Source: CAD feature listing. Evaluate the final solid. Frame: model axes, mm. Face numbers are marked on the shaded views. Give positions to 0.01 mm unless a question says otherwise; leave off trailing zeros. Write each loop counter-clockwise with the first axis right and the second up, starting at its lowest first coordinate (ties: lowest second). Pieces come first, ordered by that corner, then holes. Notation, with made-up numbers: (-3.5, -5.75) - (48.5, -5.75) arc R18 ccw to (48.5, 13.25) - close; hole circle Ø8 at (34, 41). An arc over 180 degrees is marked (long way). One line per question, with ' | ' between items. Start each with the question number.
(1) Section B-B, the plane y = 23.5. Return loops of the section in (x, z).
(2) Ray query, line 1 (X direction, y = 1, z = 0); line 2 (X direction, y = 3.4, z = 0); line 3 (X direction, y = 13, z = 0). Return the intervals inside material, ascending. Write a range as [from, to].
(3) Draft query along X for the marked faces 1, 2, 3 and 4. Return one class per face: +X half, -X half, draft (parallel to the pull), parting line (faces both ways), or undercut.
(4) Pin query (flat end, axial travel): pin 1 (2 mm diameter, centred on y = 5.5, z = 20.5, fed in from -X); pin 2 (12 mm diameter, centred on x = 16, z = -14, fed in from +Y) (3 decimals); pin 3 (6.5 mm diameter, centred on x = 17.5, z = -1.5, fed in from +Y). Return the tip coordinate at first contact, or that it passes through.
(5) Section C-C, the plane y = 5. Return loops of the section in (x, z).
```python
from build123d import *

# Parameters (mm, degrees)
SKETCH1_R           = 25
SKETCH1_R_2         = 1.8
SKETCH1_R_3         = 5.5
BOSS_EXTRUDE1_DEPTH = 7.5
SKETCH2_R           = 4
CUT_EXTRUDE1_DEPTH  = 6
SKETCH3_R           = 33
SKETCH3_R_2         = 23
BOSS_EXTRUDE2_DEPTH = 35.5
FILLET1_R           = 5


with BuildPart() as part:
    # Sketch1 → Boss-Extrude1 (new body)
    with BuildSketch(Plane(origin=(0, 0, 0), x_dir=(1, 0, 0), z_dir=(0, 1, 0))):
        with Locations(Location((0, 0, 0), (0, 0, 270))):
            Circle(SKETCH1_R)
        with Locations(Location((-19, 0, 0), (0, 0, 270))):
            Circle(SKETCH1_R_2, mode=Mode.SUBTRACT)
        with Locations(Location((19, 0, 0), (0, 0, 90))):
            Circle(SKETCH1_R_2, mode=Mode.SUBTRACT)
        with Locations(Location((0, 0, 0), (0, 0, 270))):
            Circle(SKETCH1_R_3, mode=Mode.SUBTRACT)
    extrude(amount=BOSS_EXTRUDE1_DEPTH)

    # Sketch2 → Cut-Extrude1 (cut)
    with BuildSketch(Plane(origin=(0, 7.5, 0), x_dir=(1, 0, 0), z_dir=(0, 1, 0))):
        with Locations(Location((-19, 0, 0), (0, 0, 270))):
            Circle(SKETCH2_R)
        with Locations(Location((19, 0, 0), (0, 0, 270))):
            Circle(SKETCH2_R)
    extrude(amount=-CUT_EXTRUDE1_DEPTH, mode=Mode.SUBTRACT)

    # Sketch3 → Boss-Extrude2 (add)
    with BuildSketch(Plane.XZ):
        with Locations(Location((0, 0, 0), (0, 0, 270))):
            Circle(SKETCH3_R)
        with Locations(Location((0, 0, 0), (0, 0, 270))):
            Circle(SKETCH3_R_2, mode=Mode.SUBTRACT)
    extrude(amount=-BOSS_EXTRUDE2_DEPTH)

    # Fillet1
    fillet1_edges = [part.edges().sort_by_distance(p)[0] for p in [
        (0, 35.5, 33),
        (0, 35.5, 23),
    ]]
    fillet(fillet1_edges, radius=FILLET1_R - 0.0001)  # a hair under: the kernel refuses the full size


solid = part.part
```
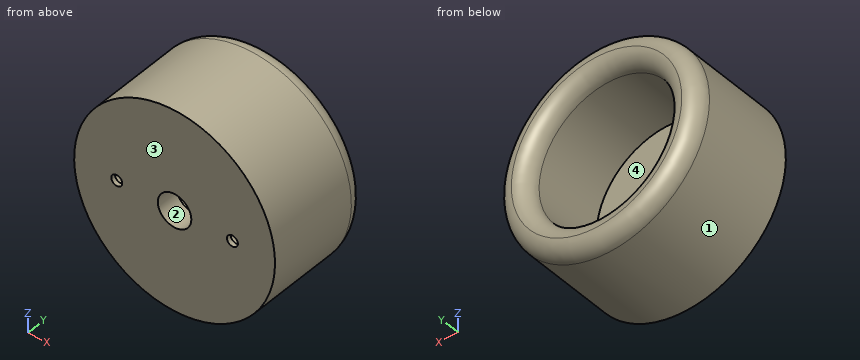
Check sheet entries:
1) outline: circle Ø66 at (0, 0); hole circle Ø46 at (0, 0)
2) line 1: [-33, -20.8], [-17.2, -5.5], [5.5, 17.2], [20.8, 33] | line 2: [-33, -23], [-15, -5.5], [5.5, 15], [23, 33] | line 3: [-33, -23], [23, 33]
3) face 1: parting line | face 2: undercut | face 3: draft | face 4: undercut
4) pin 1: x = -26.62 | pin 2: y = 35.445 | pin 3: y = 7.5
5) outline: circle Ø66 at (0, 0); hole circle Ø8 at (-19, 0); hole circle Ø11 at (0, 0); hole circle Ø8 at (19, 0)
